from build123d import *

# Parameters (mm, degrees)
SKETCH1_W      = 450
SKETCH1_H      = 300
EXTRUDE1_DEPTH = 5
EXTRUDE2_REACH = 272.463
SKETCH2_R      = 6
EXTRUDE3_REACH = 272.463
SKETCH3_W      = 10
SKETCH3_H      = 5


with BuildPart() as part:
    # Sketch1 → Extrude1 (new body)
    with BuildSketch(Plane(origin=(0, 0, 0), x_dir=(1, 0, 0), z_dir=(0, 1, 0))):
        Rectangle(SKETCH1_W, SKETCH1_H)
    extrude(amount=-EXTRUDE1_DEPTH)

    # Sketch2 → Extrude2 (cut, up to next)
    with BuildSketch(Plane(origin=(0, 0, 0), x_dir=(1, 0, 0), z_dir=(0, 1, 0)), mode=Mode.PRIVATE) as extrude2_sk1:
        with Locations(Location((0, -74.5, 0), (0, 0, 270))):
            Circle(SKETCH2_R)
    extrude2_tool1 = extrude(extrude2_sk1.sketch, amount=-EXTRUDE2_REACH, mode=Mode.PRIVATE) & part.part
    # Sketch2 → Extrude2 (cut, up to next)
    with BuildSketch(Plane(origin=(0, 0, 0), x_dir=(1, 0, 0), z_dir=(0, 1, 0)), mode=Mode.PRIVATE) as extrude2_sk2:
        with Locations(Location((118, 74.5, 0), (0, 0, 270))):
            Circle(SKETCH2_R)
    extrude2_tool2 = extrude(extrude2_sk2.sketch, amount=-EXTRUDE2_REACH, mode=Mode.PRIVATE) & part.part
    # Sketch2 → Extrude2 (cut, up to next)
    with BuildSketch(Plane(origin=(0, 0, 0), x_dir=(1, 0, 0), z_dir=(0, 1, 0)), mode=Mode.PRIVATE) as extrude2_sk3:
        with Locations(Location((-118, 74.5, 0), (0, 0, 270))):
            Circle(SKETCH2_R)
    extrude2_tool3 = extrude(extrude2_sk3.sketch, amount=-EXTRUDE2_REACH, mode=Mode.PRIVATE) & part.part
    add(extrude2_tool1.solids().sort_by_distance((0, 0, 74.5))[0], mode=Mode.SUBTRACT)
    add(extrude2_tool2.solids().sort_by_distance((118, 0, -74.5))[0], mode=Mode.SUBTRACT)
    add(extrude2_tool3.solids().sort_by_distance((-118, 0, -74.5))[0], mode=Mode.SUBTRACT)

    # Sketch3 → Extrude3 (cut, up to next)
    with BuildSketch(Plane(origin=(0, 0, 0), x_dir=(1, 0, 0), z_dir=(0, 1, 0)), mode=Mode.PRIVATE) as extrude3_sk1:
        with Locations((-105, 132.5)):
            Rectangle(SKETCH3_W, SKETCH3_H)
    extrude3_tool1 = extrude(extrude3_sk1.sketch, amount=-EXTRUDE3_REACH, mode=Mode.PRIVATE) & part.part
    # Sketch3 → Extrude3 (cut, up to next)
    with BuildSketch(Plane(origin=(0, 0, 0), x_dir=(1, 0, 0), z_dir=(0, 1, 0)), mode=Mode.PRIVATE) as extrude3_sk2:
        with Locations((105, 132.5)):
            Rectangle(SKETCH3_W, SKETCH3_H)
    extrude3_tool2 = extrude(extrude3_sk2.sketch, amount=-EXTRUDE3_REACH, mode=Mode.PRIVATE) & part.part
    add(extrude3_tool1.solids().sort_by_distance((-105, 0, -132.5))[0], mode=Mode.SUBTRACT)
    add(extrude3_tool2.solids().sort_by_distance((105, 0, -132.5))[0], mode=Mode.SUBTRACT)


solid = part.part
The listing builds one solid part. Answer for the finished solid, in the listing's coordinates (mm). Coordinates: 2 decimals unless noted, no trailing zeros. Write each loop counter-clockwise with the first axis right and the second up, starting at its lowest first coordinate (ties: lowest second). Pieces come first, ordered by that corner, then holes. Notation, with made-up numbers: M 53,54.25 L 97,54.25 A13 ccw 97,68.25 Z; hole C 66.5,34.25 d2. An arc over 180 degrees is marked long. Use one line per item in the form item = value.
Item 1: The mould has two halves that part along X. Classify faces 1 (the face through (-113.94, -2.46, -78.92)), 2 (the face through (0.264, -2.465, 68.506)), 3 (the face through (-3, -5, -2)): released by +X, released by -X, zero draft, split by the parting line, or undercut.
Model answer:
face_1 = undercut
face_2 = undercut
face_3 = zero draft
Item 2: Find section C-C, the plane z = -74.5. Give the vertices of the cut face in (x, y), plus the area to 3 significant figures.
Model answer:
outline = M -225,-5 L -124,-5 L -124,0 L -225,0 Z; M -112,-5 L 112,-5 L 112,0 L -112,0 Z; M 124,-5 L 225,-5 L 225,0 L 124,0 Z
area = 2,130 mm2
Item 3: Find section B-B, the plane z = 74.5. Give the vertices of the cut face in (x, y), plus the area to 3 significant figures.
Model answer:
outline = M -225,-5 L -6,-5 L -6,0 L -225,0 Z; M 6,-5 L 225,-5 L 225,0 L 6,0 Z
area = 2,190 mm2
Item 4: Find the intervals of material crossed by probe 1 along X at (y, z) = (-2.75, -74.5); probe 2 along Z at (x, y) = (108, -0.85); probe 3 along X at (y, z) = (-2.5, 74.5), in increasing order.
Model answer:
probe_1 = -225 to -124, -112 to 112, 124 to 225
probe_2 = -150 to -135, -130 to 150
probe_3 = -225 to -6, 6 to 225
Item 5: Find section A-A, the plane x = 118. Give the vertices of the cut face in (y, z).
Model answer:
outline = M -5,-150 L 0,-150 L 0,-80.5 L -5,-80.5 Z; M -5,-68.5 L 0,-68.5 L 0,150 L -5,150 Z
